Check sheet for the modelled part. Datum: model origin and axes. Units: mm. A direction names the side the tool comes from. Give positions to 0.01 mm unless a question says otherwise; leave off trailing zeros. Order: outer loops, then holes, each group sorted by start corner. A loop starts at its lowest first (then second) coordinate and runs counter-clockwise, first axis right, second up. Notation, with made-up numbers: M 19,-23.75 L 58,-23.75 A16 ccw 58,-12.75 Z; hole C 27.25,17 d1. An arc over 180 degrees is marked long. Return JSON: item names as keys, results as strings. Group by question number.
from build123d import *

# Parameters (mm, degrees)
SKETCH1_W           = 26
SKETCH1_H           = 47
SKETCH1_R           = 1.6
BOSS_EXTRUDE1_DEPTH = 2
FILLET1_R           = 4
SKETCH2_W           = 18
SKETCH2_H           = 35
CUT_EXTRUDE1_DEPTH  = 2
EXTRUDE_THIN1_DEPTH = 2
FILLET2_R           = 2


with BuildPart() as part:
    # Sketch1 → Boss-Extrude1 (new body)
    with BuildSketch(Plane(origin=(0, 0, 0), x_dir=(1, 0, 0), z_dir=(0, 1, 0))):
        with Locations((9, -19.5)):
            Rectangle(SKETCH1_W, SKETCH1_H)
        with Locations(Location((0, -39, 0), (0, 0, 270))):
            Circle(SKETCH1_R, mode=Mode.SUBTRACT)
        with Locations(Location((18, 0, 0), (0, 0, 270))):
            Circle(SKETCH1_R, mode=Mode.SUBTRACT)
        with Locations(Location((0, 0, 0), (0, 0, 270))):
            Circle(SKETCH1_R, mode=Mode.SUBTRACT)
        with Locations(Location((18, -39, 0), (0, 0, 270))):
            Circle(SKETCH1_R, mode=Mode.SUBTRACT)
    extrude(amount=BOSS_EXTRUDE1_DEPTH)

    # Fillet1
    fillet1_edges = [part.edges().sort_by_distance(p)[0] for p in [
        (-4, 1, -4),
        (22, 1, -4),
        (22, 1, 43),
        (-4, 1, 43),
    ]]
    fillet(fillet1_edges, radius=FILLET1_R)

    # Sketch2 → Cut-Extrude1 (cut)
    with BuildSketch(Plane(origin=(0, 2, 0), x_dir=(1, 0, 0), z_dir=(0, 1, 0))):
        with Locations((9, -19.5)):
            Rectangle(SKETCH2_W, SKETCH2_H)
    extrude(amount=-CUT_EXTRUDE1_DEPTH, mode=Mode.SUBTRACT)

    # Sketch3 → Extrude-Thin1 (add)
    with BuildSketch(Plane(origin=(0, 2, 0), x_dir=(1, 0, 0), z_dir=(0, 1, 0))):
        Polygon((-1.333931703, -2.686022019), (16.666068297, -37.686022019), (19.333931703, -36.313977981), (1.333931703, -1.313977981), align=None)
        Polygon((16.666068297, -1.313977981), (-1.333931703, -36.313977981), (1.333931703, -37.686022019), (19.333931703, -2.686022019), align=None)
    extrude(amount=-EXTRUDE_THIN1_DEPTH)

    # Fillet2
    fillet2_edges = [part.edges().sort_by_distance(p)[0] for p in [
        (1.686743027, 1, 37),
        (16.313256973, 1, 37),
        (18, 1, 5.279778109),
        (18, 1, 33.720221891),
        (16.313256973, 1, 2),
        (1.686743027, 1, 2),
        (0, 1, 33.720221891),
        (0, 1, 5.279778109),
        (7.313256973, 1, 19.5),
        (9, 1, 16.220221891),
        (10.686743027, 1, 19.5),
        (9, 1, 22.779778109),
    ]]
    fillet(fillet2_edges, radius=FILLET2_R)


solid = part.part
1) Sectioned sample at C-C on y = 1. State how many separate pieces and enclosed holes the cut face has, then the cut area to 3 significant figures.
2) Depth check by flat-ended pin: P1, Ø1.9, axis at x = 18, z = 0, coming from the -Y side. Enter the tip coordinate at first touch or a pass-through.
3) Tool access check on faces 4 (the face through (22, 1, 20)), 5 (the face through (3.272, 1.014, 2.934)). Record the directions out of +Z, -Z, +X, -X, +Y, -Y that give a thin tool (end or side, any length) a straight path to the whole face; none if there is none.
4) Release check for a two-part mould opening along X. For faces 1 (the face through (1.08, 0.99, 37.82)), 2 (the face through (20.797, 1.014, -2.859)), 3 (the face through (-2.859, 1.014, -2.797)) record: released by +X, released by -X, zero draft, split by the parting line, or undercut.
5) Sectioned sample at B-B on z = 22. Record the boundary of the cut face in (x, y), then the cut area to 3 significant figures.
6) Material ranges on line 1 along X through (y, z) = (1.5, 39); line 2 along X through (y, z) = (0.45, 25.5); line 3 along Z through (x, y) = (12, 1.55), recorded low to high.
7) Sectioned sample at D-D on z = 38. Record the boundary of the cut face in (x, y), then the cut area to 3 significant figures.
8) Sectioned sample at A-A on z = 4. Record the boundary of the cut face in (x, y), then the cut area to 3 significant figures.
Reply:
{
 "1": {"separate pieces": "1", "enclosed holes": "8", "area": "822 mm^2"},
 "2": {"P1": "through"},
 "3": {"face 4": "+Z, -Z, +X, +Y, -Y", "face 5": "+Y, -Y"},
 "4": {"face 1": "undercut", "face 2": "released by +X", "face 3": "released by -X"},
 "5": {"outline": "M -4,0 L 0,0 L 0,2 L -4,2 Z; M 6.03,0 L 11.97,0 L 11.97,2 L 6.03,2 Z; M 18,0 L 22,0 L 22,2 L 18,2 Z", "area": "27.9 mm^2"},
 "6": {"line 1": "-4 to -1.6, 1.6 to 16.4, 19.6 to 22", "line 2": "-4 to 0, 4.23 to 7.87, 10.13 to 13.77, 18 to 22", "line 3": "-4 to 2, 10.39 to 16.95, 22.05 to 28.61, 37 to 43"},
 "7": {"outline": "M -4,0 L -1.25,0 L -1.25,2 L -4,2 Z; M 1.25,0 L 16.75,0 L 16.75,2 L 1.25,2 Z; M 19.25,0 L 22,0 L 22,2 L 19.25,2 Z", "area": "42.0 mm^2"},
 "8": {"outline": "M -4,0 L 2.96,0 L 2.96,2 L -4,2 Z; M 15.04,0 L 22,0 L 22,2 L 15.04,2 Z", "area": "27.9 mm^2"}
}
